Part model, mm, in its own coordinate system. A direction names the side the tool comes from. Coordinates: 2 decimals unless noted, no trailing zeros. Write each loop counter-clockwise with the first axis right and the second up, starting at its lowest first coordinate (ties: lowest second). Pieces come first, ordered by that corner, then holes. Notation, with made-up numbers: (-8.75, 0.25) - (49.25, 0.25) arc R17 cw to (49.25, 16.25) - close; hole circle Ø8 at (78.25, 72). An arc over 180 degrees is marked (long way). Use one line per item in the form item = value. Start each with the question number.
Autodesk Fusion 360 part; units mm, degrees
sketch "Sketch1" plane through (0, 0, 0) normal (0, 0, 1) x (1, 0, 0)
  line L0 (50, 40) -> (-50, 40)
  line L1 (-50, 40) -> (-50, -20)
  line L2 (-30, -40) -> (50, -40)
  line L3 (50, -40) -> (50, 40)
  line L4 (-50, -20) -> (-30, -40)
  line L5 (-50, 40) -> (-50, 30)
  line L6 (-50, 30) -> (-30, 30)
  line L7 (-30, 30) -> (0, 0)
  line L8 (30, 0) -> (30, 40)
  line L9 (30, -30) -> (40, -40)
  line L10 (30, 0) -> (30, -30)
  line L11 (0, 0) -> (30, 0)
extrude "Extrude1" add sketch "Sketch1" along normal blind 60 contours L0 L2 L3 L8 L9 L10
extrude "Extrude2" add sketch "Sketch1" along normal blind 50 contours L0 L1 L5 L6 L7 L8 L11
extrude "Extrude3" add sketch "Sketch1" along normal blind 35 contours L1 L2 L4 L6 L7 L9 L10 L11
sketch "Sketch4" plane through (0, 0, 50) normal (0, 0, 1) x (-1, 0, 0)
  line L0 (0, 0) -> (-30, 0)
  line L1 (-30, 0) -> (-30, -40)
  line L2 (-30, -40) -> (50, -40)
  line L3 (50, -40) -> (50, -30)
  line L4 (50, -30) -> (30, -30)
  line L5 (30, -30) -> (0, 0)
  circle A0 centre (-15, -20) radius 5
sketch "Sketch5" plane through (30, 0, 0) normal (-1, 0, 0) x (0, -1, 0)
  line L0 (0, 35) -> (30, 35)
  line L1 (30, 35) -> (30, 60)
  line L2 (30, 60) -> (-40, 60)
  line L3 (-40, 60) -> (-40, 50)
  line L4 (-40, 50) -> (0, 50)
  line L5 (0, 50) -> (0, 35)
  circle A0 centre (15, 50) radius 5
extrude "Extrude4" cut sketch "Sketch4" against normal blind 50 contours A0
extrude "Extrude5" cut sketch "Sketch5" against normal blind 20 contours A0
Q1. Mould opens along Y. For faces 4 (the cylindrical face through (16.08, 24.88, 25.35)), 5 (the flat face through (50, -1, 30)), 6 (the cylindrical face through (40, -18, 54)), 7 (the flat face through (-40, 30, 42)) say: released by +Y, released by -Y, zero draft, split by the parting line, or undercut.
Q2. Which spindle directions (+Z, -Z, +X, -X, +Y, -Y) get a long thin tool onto all of the face, cutting with end or side? Do faces 1 (the flat face through (-15, 15, 42)), 2 (the flat face through (-40, -30, 17)), 3 (the flat face through (-2, 25, 50)). Say none if no direction does.
Q3. Slice it at D-D (x = 15). List the corners of the cut face in (y, z).
Q4. Drill centre lines: probe 1 along Y at (x, z) = (15, 22); probe 2 along X at (y, z) = (20, 25); probe 3 along X at (y, z) = (20, 37). Where is each one in solid material? Low to high.
Q5. Pin check, flat tips, straight feed: P1, Ø12, axis at x = 15.5, z = 52, coming from the -Y side; P2, Ø5, axis at x = 17, y = 5.5, coming from the +Z side; P3, Ø4.5, axis at x = -43, z = 40.5, coming from the -Y side. Stop position of each tip, or through.
Q6. Slice it at A-A (x = 33.5). List the corners of the cut face in (y, z), plus the area to 3 significant figures.
Q7. Slice it at C-C (y = 20). List the corners of the cut face in (x, z), plus the area to 3 significant figures.
Q8. Slice it at B-B (z = 14). List the corners of the cut face in (x, y).
Solution:
q1.face_4 = undercut
q1.face_5 = zero draft
q1.face_6 = undercut
q1.face_7 = released by -Y
q2.face_1 = +Z, -X, -Y
q2.face_2 = +Z, -Z, -X, -Y
q2.face_3 = +Z, -X, +Y, -Y
q3.outline = (-40, 0) - (15, 0) - (15, 50) - (0, 50) - (0, 35) - (-40, 35) - close; (25, 0) - (40, 0) - (40, 50) - (25, 50) - close
q4.probe_1 = -40 to 15, 25 to 40
q4.probe_2 = -50 to 10, 20 to 50
q4.probe_3 = -20 to 10, 20 to 50
q5.P1 = 0
q5.P2 = 50
q5.P3 = 30
q6.outline = (-40, 0) - (40, 0) - (40, 60) - (-33.5, 60) - (-33.5, 35) - (-40, 35) - close; hole circle Ø10 at (-15, 50)
q6.area = 4,560 mm2
q7.outline = (-50, 0) - (10, 0) - (10, 50) - (-20, 50) - (-20, 35) - (-50, 35) - close; (20, 0) - (50, 0) - (50, 60) - (30, 60) - (30, 50) - (20, 50) - close
q7.area = 4,250 mm2
q8.outline = (-50, -20) - (-30, -40) - (50, -40) - (50, 40) - (-50, 40) - close; hole circle Ø10 at (15, 20)
